Verification items for the finished model (mm, model axes). Round coordinates to 2 decimals unless told otherwise and drop trailing zeros. Write each loop counter-clockwise with the first axis right and the second up, starting at its lowest first coordinate (ties: lowest second). Pieces come first, ordered by that corner, then holes. Notation, with made-up numbers: M 78,15 L 135,15 A23 cw 135,43 Z; hole C 32,-34.75 d9. An arc over 180 degrees is marked long. Answer in a Markdown table with one row per item. Add a question column.
1. Sectioned sample at A-A on x = 72. Record the cut outline in (y, z), plus the area to 3 significant figures.
2. Go/stop test with a flat-tipped pin: pin 1 Ø3.5 at (x, z) = (15, -40) entering from -Y (3 decimals). Record where the tip stops, or that it passes through.
3. Sectioned sample at D-D on x = 15. Record the cut outline in (y, z).
4. Sectioned sample at C-C on z = -40. Record the cut outline in (x, y).
5. Sectioned sample at B-B on y = 3.75. Record the cut outline in (x, z), plus the area to 3 significant figures.
6. Material ranges on probe 1 along X at (y, z) = (4.75, -40); probe 2 along Z at (x, y) = (70, 4.6); probe 3 along X at (y, z) = (4.05, -41), recorded low to high.
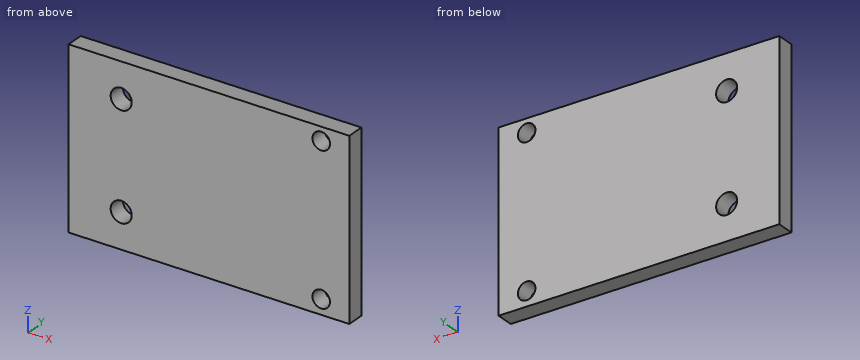
```python
from build123d import *

# Parameters (mm, degrees)
SKETCH1_W           = 80
SKETCH1_H           = 50
SKETCH1_R           = 3
BOSS_EXTRUDE1_DEPTH = 5
SKETCH2_R           = 2.5
CUT_EXTRUDE1_DEPTH  = 10


with BuildPart() as part:
    # Sketch1 → Boss-Extrude1 (new body)
    with BuildSketch(Plane(origin=(0, 0, 0), x_dir=(1, 0, 0), z_dir=(0, 1, 0))):
        with Locations((40, 25)):
            Rectangle(SKETCH1_W, SKETCH1_H)
        with Locations(Location((15, 40, 0), (0, 0, 270))):
            Circle(SKETCH1_R, mode=Mode.SUBTRACT)
        with Locations(Location((15, 10, 0), (0, 0, 270))):
            Circle(SKETCH1_R, mode=Mode.SUBTRACT)
    extrude(amount=BOSS_EXTRUDE1_DEPTH)

    # Sketch2 → Cut-Extrude1 (cut)
    with BuildSketch(Plane(origin=(0, 5, 0), x_dir=(1, 0, 0), z_dir=(0, 1, 0))):
        with Locations(Location((72, 3.828026959, 0), (0, 0, 270))):
            Circle(SKETCH2_R)
        with Locations(Location((72, 45.828026959, 0), (0, 0, 270))):
            Circle(SKETCH2_R)
    extrude(amount=-CUT_EXTRUDE1_DEPTH, mode=Mode.SUBTRACT)


solid = part.part
```
Geometry check:
| question | item | result |
|---|---|---|
| 1 | outline | M 0,-50 L 5,-50 L 5,-48.33 L 0,-48.33 Z; M 0,-43.33 L 5,-43.33 L 5,-6.33 L 0,-6.33 Z; M 0,-1.33 L 5,-1.33 L 5,0 L 0,0 Z |
| 1 | area | 200 mm2 |
| 2 | pin 1 | passes through |
| 3 | outline | M 0,-50 L 5,-50 L 5,-43 L 0,-43 Z; M 0,-37 L 5,-37 L 5,-13 L 0,-13 Z; M 0,-7 L 5,-7 L 5,0 L 0,0 Z |
| 4 | outline | M 0,0 L 12,0 L 12,5 L 0,5 Z; M 18,0 L 80,0 L 80,5 L 18,5 Z |
| 5 | outline | M 0,-50 L 80,-50 L 80,0 L 0,0 Z; hole C 15,-40 d6; hole C 15,-10 d6; hole C 72,-45.83 d5; hole C 72,-3.83 d5 |
| 5 | area | 3,900 mm2 |
| 6 | probe 1 | x = 0 to 12, 18 to 80 |
| 6 | probe 2 | z = -50 to -47.33, -44.33 to -5.33, -2.33 to 0 |
| 6 | probe 3 | x = 0 to 12.17, 17.83 to 80 |
